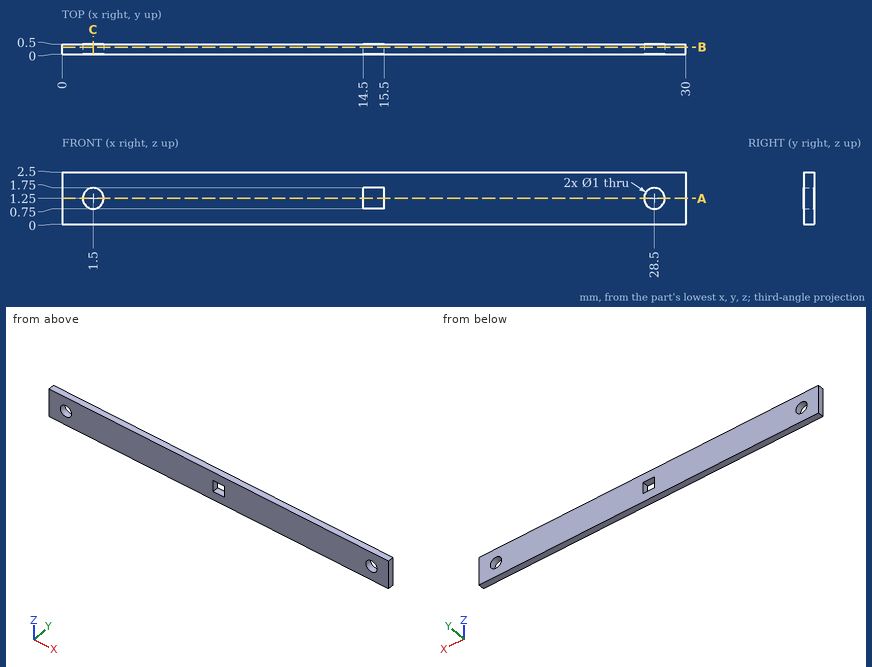
Answer from the drawing. Dimensions are ordinates in mm from the lowest x, y and z of the part. Coordinates: 2 decimals unless noted, no trailing zeros. Order: outer loops, then holes, each group sorted by start corner. A loop starts at its lowest first (then second) coordinate and runs counter-clockwise, first axis right, second up. Notation, with made-up numbers: (-15, 10) -> (29, 10) arc R21 ccw to (29, 24) -> close; hole circle Ø1 at (56, 86.25). An arc over 180 degrees is marked (long way). Answer as a JSON object with one key per item and string values.
1) A cutting plane is placed at C-C, the plane x = 1.5. Determine the outline of the cut face in (y, z).
Model answer:
{"outline": "(0, 0) -> (0.5, 0) -> (0.5, 0.75) -> (0, 0.75) -> close; (0, 1.75) -> (0.5, 1.75) -> (0.5, 2.5) -> (0, 2.5) -> close"}
2) A cutting plane is placed at B-B, the plane y = 0.35. Determine the outline of the cut face in (x, z), plus the area to 3 significant figures.
Model answer:
{"outline": "(0, 0) -> (30, 0) -> (30, 2.5) -> (0, 2.5) -> close; hole circle Ø1 at (1.5, 1.25); hole (14.5, 0.75) -> (15.5, 0.75) -> (15.5, 1.75) -> (14.5, 1.75) -> close; hole circle Ø1 at (28.5, 1.25)", "area": "72.4 mm²"}
3) Consider line 1 along X through (y, z) = (0.2, 1.2); line 2 along X through (y, z) = (0.1, 1.6); line 3 along Z through (x, y) = (1.5, 0.4). Determine where each line is inside the solid, lowest interval first. Write a range as from..to.
Model answer:
{"line 1": "x = 0..1, 2..14.5, 15.5..28, 29..30", "line 2": "x = 0..1.14, 1.86..14.5, 15.5..28.14, 28.86..30", "line 3": "z = 0..0.75, 1.75..2.5"}
4) A cutting plane is placed at A-A, the plane z = 1.25. Determine the outline of the cut face in (x, y).
Model answer:
{"outline": "(0, 0) -> (1, 0) -> (1, 0.5) -> (0, 0.5) -> close; (2, 0) -> (14.5, 0) -> (14.5, 0.5) -> (2, 0.5) -> close; (15.5, 0) -> (28, 0) -> (28, 0.5) -> (15.5, 0.5) -> close; (29, 0) -> (30, 0) -> (30, 0.5) -> (29, 0.5) -> close"}
